Design review of the part built by this model. Coordinates are the model's own, in mm. A direction names the side the tool comes from. Give positions to 0.01 mm unless a question says otherwise; leave off trailing zeros. Loops run counter-clockwise (first coordinate to the right, second up) from the corner with the lowest first, then second, coordinate; pieces in that order, holes last. Notation, with made-up numbers: M -4,41 L 11,41 A25 ccw 11,65 Z; hole C 1.5,36.5 d6. An arc over 180 degrees is marked long. Use a Markdown table: item, result. Add a question column.
(1) For probe 1 along X at (y, z) = (7.25, -1.5); probe 2 along Y at (x, z) = (3.75, -1.5); probe 3 along Y at (x, z) = (-2.5, -1.5), list the stretches that pass through material, from the lowest coordinate up.
(2) Add section B-B, the plane z = 3. Give the boundary of the cut face in (x, y).
(3) Add section C-C, the plane y = -0.25. Give the boundary of the cut face in (x, z), then the cut area to 3 significant figures.
(4) Add section D-D, the plane x = 6. Give the boundary of the cut face in (y, z).
(5) For faces 5 (the face through (6.873, 3, 1)), 6 (the face through (-2, 0, 1)), 7 (the face through (3, 9, -3.535)), list the 3-axis set-ups (+Z, -Z, +X, -X, +Y, -Y) from which the entire face can be reached by the end or side of a thin tool; tool diameter is ignored.
(6) Add section A-A, the plane y = 2.25. Give the boundary of the cut face in (x, z), then the cut area to 3 significant figures.
(7) Draft analysis for pull direction X (two halves, no side actions). For faces 1 (the face through (3, 9, 6.465)), 2 (the face through (8.873, 4, 1)), 3 (the face through (-3.127, 5, 2)), 4 (the face through (-1.127, 4, 2)), state which applies: pulls with the +X half, pulls with the -X half, needs draft (parallel to the pull), parting line crosses it, or undercut.
(8) Insertion check: pin 1 Ø6 at (x, z) = (1.5, -1) entering from -Y; pin 2 Ø1.5 at (x, z) = (1.5, 5) entering from -Y. Each pin has a flat end and moves straight along its axis. Give the tip position at first contact, or say it passes through.
```python
from build123d import *

# Parameters (mm, degrees)
SKETCH1_W           = 2
SKETCH1_H           = 10
BOSS_EXTRUDE1_DEPTH = 10
SKETCH2_W           = 10
SKETCH2_H           = 2
BOSS_EXTRUDE2_DEPTH = 10
SKETCH3_W           = 2
SKETCH3_H           = 10
BOSS_EXTRUDE3_DEPTH = 10


with BuildPart() as part:
    # Sketch1 → Boss-Extrude1 (new body)
    with BuildSketch(Plane(origin=(0, 0, 0), x_dir=(1, 0, 0), z_dir=(0, 1, 0))):
        with Locations((-2.126760563, -1.464788732)):
            Rectangle(SKETCH1_W, SKETCH1_H)
    extrude(amount=BOSS_EXTRUDE1_DEPTH)

    # Sketch2 → Boss-Extrude2 (add)
    with BuildSketch(Plane(origin=(-1.126760563, 0, 0), x_dir=(0, 0, -1), z_dir=(1, 0, 0))):
        with Locations((-1.464788732, 9)):
            Rectangle(SKETCH2_W, SKETCH2_H)
    extrude(amount=BOSS_EXTRUDE2_DEPTH)

    # Sketch3 → Boss-Extrude3 (add)
    with BuildSketch(Plane.XZ.offset(-8)):
        with Locations((7.873239437, 1.464788732)):
            Rectangle(SKETCH3_W, SKETCH3_H)
    extrude(amount=BOSS_EXTRUDE3_DEPTH)


solid = part.part
```
Established:
| question | item | result |
|---|---|---|
| 1 | probe 1 | -3.13 to -1.13, 6.87 to 8.87 |
| 1 | probe 2 | 8 to 10 |
| 1 | probe 3 | 0 to 10 |
| 2 | outline | M -3.13,0 L -1.13,0 L -1.13,8 L 6.87,8 L 6.87,-2 L 8.87,-2 L 8.87,10 L -3.13,10 Z |
| 3 | outline | M 6.87,-3.54 L 8.87,-3.54 L 8.87,6.46 L 6.87,6.46 Z |
| 3 | area | 20.0 mm^2 |
| 4 | outline | M 8,-3.54 L 10,-3.54 L 10,6.46 L 8,6.46 Z |
| 5 | face 5 | +Z, -Z, -Y |
| 5 | face 6 | +Z, -Z, -X, -Y |
| 5 | face 7 | -Z, +X, -X, +Y, -Y |
| 6 | outline | M -3.13,-3.54 L -1.13,-3.54 L -1.13,6.46 L -3.13,6.46 Z; M 6.87,-3.54 L 8.87,-3.54 L 8.87,6.46 L 6.87,6.46 Z |
| 6 | area | 40.0 mm^2 |
| 7 | face 1 | needs draft |
| 7 | face 2 | pulls with the +X half |
| 7 | face 3 | pulls with the -X half |
| 7 | face 4 | undercut |
| 8 | pin 1 | y = 0 |
| 8 | pin 2 | y = 8 |
